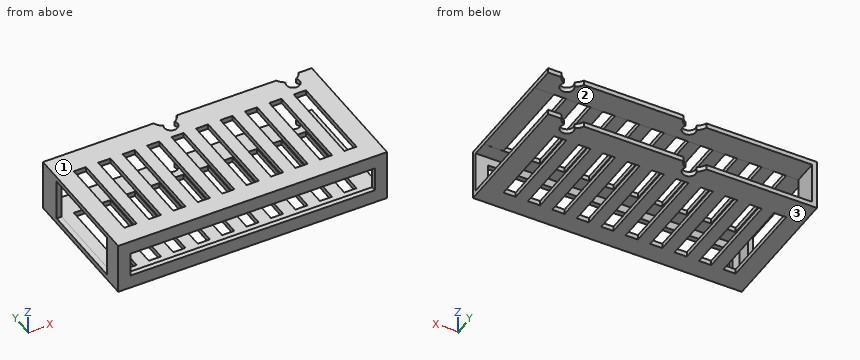
```python
from build123d import *

# Parameters (mm, degrees)
SKETCH_1_W           = 110
SKETCH_1_H           = 21
EXTRUDE_1_DEPTH      = 55
SHELL_1_T            = -2
SKETCH_2_W           = 17
SKETCH_2_H           = 53
CUT_EXTRUDE_1_DEPTH  = 50
SKETCH_8_W           = 5
SKETCH_8_H           = 37
CUT_EXTRUDE_8_DEPTH  = 22
SKETCH_9_W           = 16.817883905
SKETCH_9_H           = 37
CUT_EXTRUDE_9_DEPTH  = 111
SKETCH_10_W          = 100
SKETCH_10_H          = 10
CUT_EXTRUDE_10_DEPTH = 56
CUT_EXTRUDE_11_DEPTH = 22


with BuildPart() as part:
    # 草图1 → 凸台-拉伸1 (new body)
    with BuildSketch(Plane(origin=(0, 0, 0), x_dir=(1, 0, 0), z_dir=(0, 1, 0))):
        Rectangle(SKETCH_1_W, SKETCH_1_H)
    extrude(amount=EXTRUDE_1_DEPTH)

    # 抽壳1
    shell_1_openings = [part.faces().sort_by_distance(p)[0] for p in [
        (0, 55, 0),
    ]]
    offset(amount=SHELL_1_T, openings=shell_1_openings, kind=Kind.INTERSECTION)

    # 草图2 → 切除-拉伸1 (cut)
    with BuildSketch(Plane(origin=(55, 0, 0), x_dir=(0, 0, -1), z_dir=(1, 0, 0))):
        with Locations((0, 28.5)):
            Rectangle(SKETCH_2_W, SKETCH_2_H)
    extrude(amount=-CUT_EXTRUDE_1_DEPTH, mode=Mode.SUBTRACT)

    # 草图8 → 切除-拉伸8 (cut, through all)
    with BuildSketch(Plane(origin=(0, 0, -10.5), x_dir=(-1, 0, 0), z_dir=(0, 0, -1))):
        with Locations((-34.5, 26.5)):
            Rectangle(SKETCH_8_W, SKETCH_8_H)
        with Locations((-44.5, 26.5)):
            Rectangle(SKETCH_8_W, SKETCH_8_H)
        with Locations((-24.5, 26.5)):
            Rectangle(SKETCH_8_W, SKETCH_8_H)
        with Locations((-14.5, 26.5)):
            Rectangle(SKETCH_8_W, SKETCH_8_H)
        with Locations((-4.5, 26.5)):
            Rectangle(SKETCH_8_W, SKETCH_8_H)
        with Locations((5.5, 26.5)):
            Rectangle(SKETCH_8_W, SKETCH_8_H)
        with Locations((15.5, 26.5)):
            Rectangle(SKETCH_8_W, SKETCH_8_H)
        with Locations((25.5, 26.5)):
            Rectangle(SKETCH_8_W, SKETCH_8_H)
        with Locations((35.5, 26.5)):
            Rectangle(SKETCH_8_W, SKETCH_8_H)
        with Locations((45.5, 26.5)):
            Rectangle(SKETCH_8_W, SKETCH_8_H)
    extrude(amount=-CUT_EXTRUDE_8_DEPTH, mode=Mode.SUBTRACT)

    # 草图9 → 切除-拉伸9 (cut, through all)
    with BuildSketch(Plane.ZY.offset(55)):
        with Locations((0.111623124, 26.5)):
            Rectangle(SKETCH_9_W, SKETCH_9_H)
    extrude(amount=-CUT_EXTRUDE_9_DEPTH, mode=Mode.SUBTRACT)

    # 草图10 → 切除-拉伸10 (cut, through all)
    with BuildSketch(Plane.XZ):
        Rectangle(SKETCH_10_W, SKETCH_10_H)
    extrude(amount=-CUT_EXTRUDE_10_DEPTH, mode=Mode.SUBTRACT)

    # 草图5 → 切除-拉伸11 (cut, through all)
    with BuildSketch(Plane(origin=(0, 0, -10.5), x_dir=(-1, 0, 0), z_dir=(0, 0, -1))):
        with BuildLine():
            ThreePointArc((-47.120181843, 52.510910871), (-45, 48.139136677), (-42.879818157, 52.510910871))
            ThreePointArc((-42.879818157, 52.510910871), (-45, 62.039136677), (-47.120181843, 52.510910871))
        make_face()
        with BuildLine():
            ThreePointArc((2.675165182, 52.212141801), (5, 48.139136677), (7.324834818, 52.212141801))
            ThreePointArc((7.324834818, 52.212141801), (5, 61.638781957), (2.675165182, 52.212141801))
        make_face()
    extrude(amount=-CUT_EXTRUDE_11_DEPTH, mode=Mode.SUBTRACT)


solid = part.part
```
Work out the finished part from the listing and answer in its coordinate system (mm). Face numbers are marked on the shaded views. Give positions to 0.01 mm unless a question says otherwise; leave off trailing zeros. Loops run counter-clockwise (first coordinate to the right, second up) from the corner with the lowest first, then second, coordinate; pieces in that order, holes last. Notation, with made-up numbers: (-39.5, -28.5) -> (13.5, -28.5) arc R22 ccw to (13.5, -2.5) -> close; hole circle Ø11 at (63.5, 48.25). An arc over 180 degrees is marked (long way). Write item = value, one per line. Start each with the question number.
(1) Find section C-C on z = -6.25. Give the vertices of the cut face in (x, y).
(2) Given pin 1 Ø5 at (x, y) = (-5, 50.84) entering from -Z; pin 2 Ø11 at (x, y) = (-3, 49.5) entering from -Z, each flat-ended and moving along its own axis, determine where each tip first touches the part or whether it passes through.
(3) Find section A-A on x = 34. Give the vertices of the cut face in (y, z), and give its area (3 significant figures).
(4) Find section B-B on z = 4. Give the vertices of the cut face in (x, y).
(5) The mould has two halves that part along Z. Classify the marked faces 1, 2 and 3: +Z half, -Z half, draft (parallel to the pull), parting line (faces both ways), or undercut.
(6) Find the intervals of material crossed by probe 1 along Z at (x, y) = (-22, 52); probe 2 along Y at (x, z) = (-5, -9.9); probe 3 along Y at (x, z) = (-38.5, -7), in increasing order. Write a range as from..to.
From the geometry:
q1.outline = (-55, 0) -> (55, 0) -> (55, 2) -> (-53, 2) -> (-53, 8) -> (-55, 8) -> close; (-55, 45) -> (-53, 45) -> (-53, 55) -> (-55, 55) -> close
q2.pin_1 = through
q2.pin_2 = -10.5
q3.outline = (0, -10.5) -> (8, -10.5) -> (8, -8.5) -> (2, -8.5) -> (2, -5) -> (0, -5) -> close; (0, 5) -> (2, 5) -> (2, 8.5) -> (8, 8.5) -> (8, 10.5) -> (0, 10.5) -> close; (45, -10.5) -> (55, -10.5) -> (55, -8.5) -> (45, -8.5) -> close; (45, 8.5) -> (55, 8.5) -> (55, 10.5) -> (45, 10.5) -> close
q3.area = 86.0 mm^2
q4.outline = (-55, 0) -> (-50, 0) -> (-50, 2) -> (-53, 2) -> (-53, 8) -> (-55, 8) -> close; (-55, 45) -> (-53, 45) -> (-53, 55) -> (-55, 55) -> close; (50, 0) -> (55, 0) -> (55, 2) -> (50, 2) -> close
q5.face_1 = +Z half
q5.face_2 = undercut
q5.face_3 = -Z half
q6.probe_1 = -10.5..-8.5, 8.5..10.5
q6.probe_2 = 0..8, 45..48.14
q6.probe_3 = 0..2
